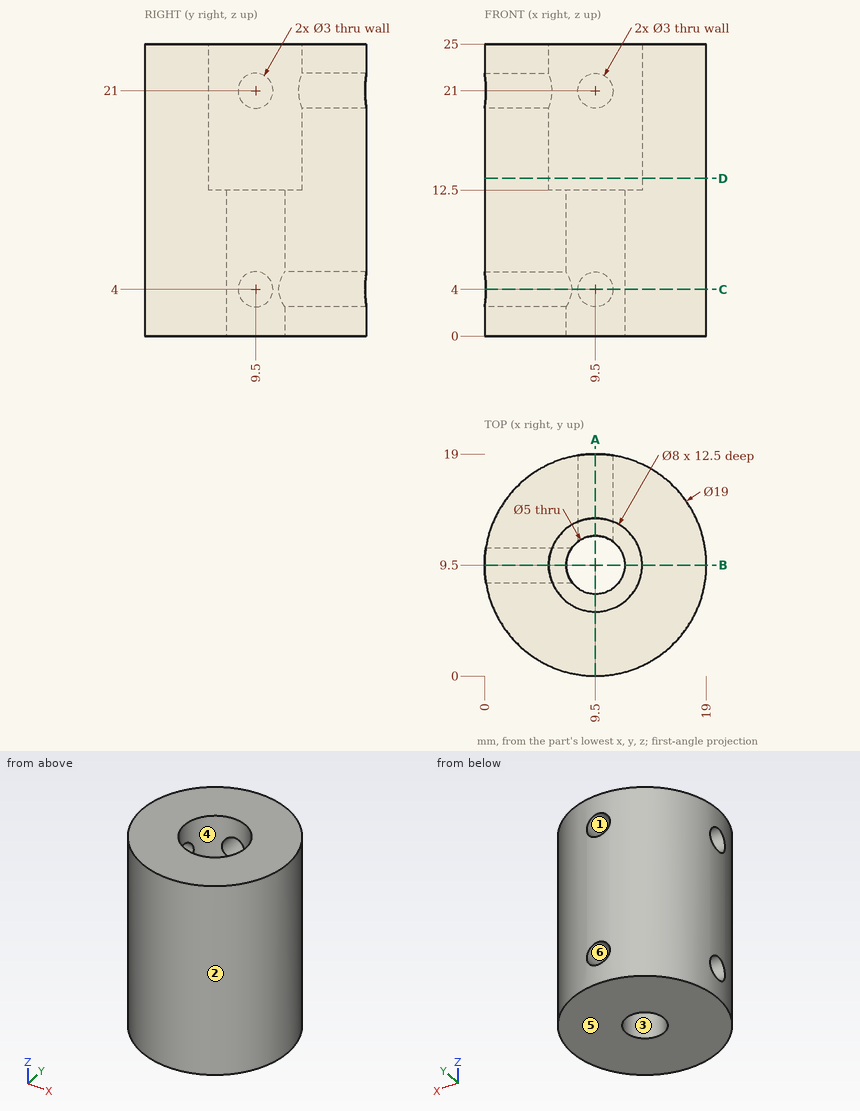
Study the drawing (mm; zero at the part's minimum x, y, z) and answer. A direction names the side the tool comes from. Coordinates: 2 decimals unless noted, no trailing zeros. Write each loop counter-clockwise with the first axis right and the second up, starting at its lowest first coordinate (ties: lowest second). Pieces come first, ordered by that corner, then holes.
Q1. Find the intervals of material crossed by line 1 along Z through (x, y) = (9.5, 14.75); line 2 along Y through (x, z) = (9.5, 8); line 3 along X through (y, z) = (9.75, 16), in increasing order.
Returned:
line 1: z = 0 to 2.5, 5.5 to 19.5, 22.5 to 25
line 2: y = 0 to 7, 12 to 19
line 3: x = 0 to 5.51, 13.49 to 19
Q2. Section C-C, the plane z = 4 is taken. Write down the section's boundary in (x, y).
Returned:
outline: (0.12, 8) arc R9.5 ccw (long way) to (11, 18.88) - (11, 11.5) arc R2.5 cw (long way) to (7.5, 8) - close; (0.12, 11) - (7.5, 11) arc R2.5 cw to (8, 11.5) - (8, 18.88) arc R9.5 ccw to start
Q3. Section A-A, the plane x = 9.5 is taken. Write down the section's boundary in (y, z).
Returned:
outline: (0, 0) - (7, 0) - (7, 12.5) - (5.5, 12.5) - (5.5, 25) - (0, 25) - close; (12, 0) - (19, 0) - (19, 2.5) - (12, 2.5) - close; (12, 5.5) - (19, 5.5) - (19, 19.5) - (13.5, 19.5) - (13.5, 12.5) - (12, 12.5) - close; (13.5, 22.5) - (19, 22.5) - (19, 25) - (13.5, 25) - close
Q4. Section B-B, the plane y = 9.5 is taken. Write down the section's boundary in (x, z), then the cut area to 3 significant figures.
Returned:
outline: (0, 0) - (7, 0) - (7, 2.5) - (0, 2.5) - close; (0, 5.5) - (7, 5.5) - (7, 12.5) - (5.5, 12.5) - (5.5, 19.5) - (0, 19.5) - close; (0, 22.5) - (5.5, 22.5) - (5.5, 25) - (0, 25) - close; (12, 0) - (19, 0) - (19, 25) - (13.5, 25) - (13.5, 12.5) - (12, 12.5) - close
area: 275 mm2
Q5. The mould has two halves that part along Y. Classify the marked faces 1, 2, 3 and 4: released by +Y, released by -Y, zero draft, split by the parting line, or undercut.
Returned:
face 1: zero draft
face 2: split by the parting line
face 3: undercut
face 4: undercut
Q6. Given P1, Ø1, axis at y = 15.5, z = 4, coming from the -X side; P2, Ø10, axis at y = 10.5, z = 20.5, coming from the +X side; P3, Ø1.5, axis at x = 13, z = 3.5, coming from the +Y side; P4, Ø1.5, axis at x = 6, z = 3.5, coming from the -Y side, each flat-ended and moving along its own axis, determine where each tip first touches the part or whether it passes through.
Returned:
P1: stops at x = 1.75
P2: stops at x = 19
P3: stops at y = 18.59
P4: stops at y = 0.41
Q7. Which of the six approach directions +Z, -Z, +X, -X, +Y, -Y give full straight-line access (tool end or side, diameter ignored) to the marked faces 5 and 6?
Returned:
face 5: -Z, +X, -X, +Y, -Y
face 6: +Y
Q8. Section D-D, the plane z = 13.5 is taken. Write down the section's boundary in (x, y), then the cut area to 3 significant figures.
Returned:
outline: circle Ø19 at (9.5, 9.5); hole circle Ø8 at (9.5, 9.5)
area: 233 mm2
